Here's how the part is built. I have some questions about the finished solid (model axes, mm). A direction names the side the tool comes from. Coordinates: 2 decimals unless noted, no trailing zeros. Write each loop counter-clockwise with the first axis right and the second up, starting at its lowest first coordinate (ties: lowest second). Pieces come first, ordered by that corner, then holes. Notation, with made-up numbers: M 38,9 L 70,9 A30 cw 70,36 Z; hole C 72.5,54.5 d3. An arc over 180 degrees is marked long. Use a Markdown table: item, result.
```python
from build123d import *

# Parameters (mm, degrees)
EXTRUDE_THIN1_DEPTH = 200
CUT_EXTRUDE1_REACH  = 210.749
SKETCH3_R           = 1.5


with BuildPart() as part:
    # Sketch2 → Extrude-Thin1 (new body)
    with BuildSketch(Plane(origin=(0, 0, 0), x_dir=(0, 0, -1), z_dir=(1, 0, 0))):
        Polygon((-2.5, 50), (-2.5, -1.035533906), (33.587572106, -37.123106012), (37.123106012, -33.587572106), (2.5, 1.035533906), (2.5, 50), align=None)
    extrude(amount=EXTRUDE_THIN1_DEPTH)

    # Sketch3 → Cut-Extrude1 (cut, up to next)
    with BuildSketch(Plane(origin=(0, 1.767766953, -1.767766953), x_dir=(1, 0, 0), z_dir=(0, 0.7071067811865489, -0.7071067811865462)), mode=Mode.PRIVATE) as cut_extrude1_sk1:
        with Locations(Location((132, 42, 0), (0, 0, 270))):
            Circle(SKETCH3_R)
    cut_extrude1_tool1 = extrude(cut_extrude1_sk1.sketch, amount=-CUT_EXTRUDE1_REACH, mode=Mode.PRIVATE) & part.part
    # Sketch3 → Cut-Extrude1 (cut, up to next)
    with BuildSketch(Plane(origin=(0, 1.767766953, -1.767766953), x_dir=(1, 0, 0), z_dir=(0, 0.7071067811865489, -0.7071067811865462)), mode=Mode.PRIVATE) as cut_extrude1_sk2:
        with Locations(Location((196, 42, 0), (0, 0, 270))):
            Circle(SKETCH3_R)
    cut_extrude1_tool2 = extrude(cut_extrude1_sk2.sketch, amount=-CUT_EXTRUDE1_REACH, mode=Mode.PRIVATE) & part.part
    add(cut_extrude1_tool1.solids().sort_by_distance((132, -27.930718, -31.466252))[0], mode=Mode.SUBTRACT)
    add(cut_extrude1_tool2.solids().sort_by_distance((196, -27.930718, -31.466252))[0], mode=Mode.SUBTRACT)


solid = part.part
```
1. We'd pull the mould along Z, two halves only. Please class faces 1 (the face through (133.487, -29.812, -29.861)), 2 (the face through (197.487, -29.812, -29.861)), 3 (the face through (200, -3, -5)), 4 (the face through (98.6, -16.518, -20.054)): +Z half, -Z half, draft (parallel to the pull), parting line (faces both ways), or undercut.
Answers follow:
| item | result |
|---|---|
| face 1 | undercut |
| face 2 | undercut |
| face 3 | draft |
| face 4 | -Z half |
2. I need wall thicknesses on probe 1 along Z at (x, y) = (99.5, 32.5); probe 2 along Y at (x, z) = (151.5, -28); probe 3 along Z at (x, y) = (38, -15). Which ranges of each line are inside material? Lowest first, please.
Answers follow:
| item | result |
|---|---|
| probe 1 | z = -2.5 to 2.5 |
| probe 2 | y = -31.54 to -24.46 |
| probe 3 | z = -18.54 to -11.46 |
3. Suppose I cut it at B-B on y = 34. Write out the boundary of the cut face in (x, z).
Answers follow:
| item | result |
|---|---|
| outline | M 0,-2.5 L 200,-2.5 L 200,2.5 L 0,2.5 Z |
4. Will these pins go through, and if not, where does the flat tip stop? pin 1 Ø6 at (x, z) = (92.5, -5.5) entering from -Y; pin 2 Ø6 at (x, y) = (152.5, 5) entering from -Z.
Answers follow:
| item | result |
|---|---|
| pin 1 | stops at y = -12.04 |
| pin 2 | stops at z = -2.5 |
5. Suppose I cut it at C-C on z = -14. Write out the boundary of the cut face in (x, y), and give its area (3 significant figures).
Answers follow:
| item | result |
|---|---|
| outline | M 0,-17.54 L 200,-17.54 L 200,-10.46 L 0,-10.46 Z |
| area | 1,410 mm2 |
6. Which directions (+Z, -Z, +X, -X, +Y, -Y) give clear straight access to the entire face, cutting with the end or side of a thin tool? Please do faces 5 (the face through (99, 25, -2.5)), 6 (the face through (98.6, -35.38, -35.33)).
Answers follow:
| item | result |
|---|---|
| face 5 | -Z, +X, -X, +Y |
| face 6 | -Z, +X, -X, -Y |
7. Suppose I cut it at A-A on x = 91.5. Write out the boundary of the cut face in (y, z), and give its area (3 significant figures).
Answers follow:
| item | result |
|---|---|
| outline | M -37.12,-33.59 L -33.59,-37.12 L 1.04,-2.5 L 50,-2.5 L 50,2.5 L -1.04,2.5 Z |
| area | 500 mm2 |
